Design review of the part built by this model. Coordinates are the model's own, in mm. A direction names the side the tool comes from. Coordinates: 2 decimals unless noted, no trailing zeros. Write each loop counter-clockwise with the first axis right and the second up, starting at its lowest first coordinate (ties: lowest second). Pieces come first, ordered by that corner, then holes. Notation, with made-up numbers: (-20.5, 72) - (29.5, 72) arc R25 cw to (29.5, 108) - close; hole circle Ø3 at (86.25, 12.5). An arc over 180 degrees is marked (long way). Use a Markdown table: item, result.
from build123d import *

# Parameters (mm, degrees)
SKETCH_W        = 37
SKETCH_H        = 37
PAD_DEPTH       = 17.8
SKETCH001_W     = 30.1
SKETCH001_H     = 30.1
POCKET_DEPTH    = 14.8
SKETCH002_R     = 1
PAD001_DEPTH    = 3.2
SKETCH003_W     = 31
SKETCH003_H     = 31
POCKET001_DEPTH = 10
SKETCH004_W     = 2.2
SKETCH004_H     = 1.6
POCKET002_DEPTH = 10
POCKET003_DEPTH = 2
POCKET004_DEPTH = 1.5
SKETCH011_W     = 8.94
SKETCH011_H     = 3.16
POCKET007_DEPTH = 3.5
SKETCH012_W     = 14.612
SKETCH012_H     = 7.87
POCKET008_DEPTH = 1.5
SKETCH013_W     = 7.7
SKETCH013_H     = 1.75
POCKET009_DEPTH = 3.5
PAD005_DEPTH    = 5
POCKET014_DEPTH = 2.1
SKETCH021_W     = 2.79
SKETCH021_H     = 4.318
POCKET013_DEPTH = 2.5
POCKET011_DEPTH = 3
POCKET012_DEPTH = 3.5
FILLET006_R     = 2
CHAMFER_SIZE    = 1
FILLET007_R     = 1
FILLET008_R     = 1


with BuildPart() as part:
    # Sketch → Pad (new body)
    with BuildSketch(Plane.XY):
        Rectangle(SKETCH_W, SKETCH_H)
    extrude(amount=PAD_DEPTH)

    # Sketch001 → Pocket (cut)
    with BuildSketch(Plane.XY):
        Rectangle(SKETCH001_W, SKETCH001_H)
    extrude(amount=POCKET_DEPTH, mode=Mode.SUBTRACT)

    # Sketch002 (on Face11 of Pocket) → Pad001 (join)
    with BuildSketch(Plane.XY.offset(14.8)):
        with Locations((1.018, 12.079)):
            Circle(SKETCH002_R)
        with Locations((9.384, -0.351)):
            Circle(SKETCH002_R)
        with Locations((-7.888, -4.939)):
            Circle(SKETCH002_R)
    extrude(amount=-PAD001_DEPTH)

    # Sketch003 → Pocket001 (cut)
    with BuildSketch(Plane.XY):
        Rectangle(SKETCH003_W, SKETCH003_H)
    extrude(amount=POCKET001_DEPTH, mode=Mode.SUBTRACT)

    # Sketch004 → Pocket002 (cut)
    with BuildSketch(Plane.XY):
        with Locations((-4.066, -15.8)):
            Rectangle(SKETCH004_W, SKETCH004_H)
    extrude(amount=POCKET002_DEPTH, mode=Mode.SUBTRACT)

    # Sketch005 (on Face16 of Pocket002) → Pocket003 (cut)
    with BuildSketch(Plane(origin=(0, -15.05, 0), x_dir=(-1, 0, 0), z_dir=(0, 1, 0))):
        with BuildLine():
            ThreePointArc((0.066, 14.4), (-2.134, 12.2), (0.066, 10))
            Line((0.066, 10), (6.566, 10))
            ThreePointArc((6.566, 10), (8.766, 12.2), (6.566, 14.4))
            Line((6.566, 14.4), (0.066, 14.4))
        make_face()
    extrude(amount=-POCKET003_DEPTH, mode=Mode.SUBTRACT)

    # Sketch006 (on Face18 of Pocket003) → Pocket004 (cut)
    with BuildSketch(Plane(origin=(0, -17.05, 0), x_dir=(-1, 0, 0), z_dir=(0, 1, 0))):
        with BuildLine():
            ThreePointArc((2.566, 14.3), (0.466, 12.2), (2.566, 10.1))
            Line((2.566, 10.1), (4.066, 10.1))
            ThreePointArc((4.066, 10.1), (6.166, 12.2), (4.066, 14.3))
            Line((4.066, 14.3), (2.566, 14.3))
        make_face()
    extrude(amount=-POCKET004_DEPTH, mode=Mode.SUBTRACT)

    # Sketch011 (on Face26 of Pocket004) → Pocket007 (cut)
    with BuildSketch(Plane.XZ.offset(-15.05)):
        with Locations((9.638, 13.18)):
            Rectangle(SKETCH011_W, SKETCH011_H)
    extrude(amount=-POCKET007_DEPTH, mode=Mode.SUBTRACT)

    # Sketch012 (on Face1 of Pocket007) → Pocket008 (cut)
    with BuildSketch(Plane(origin=(0, 18.5, 0), x_dir=(-1, 0, 0), z_dir=(0, 1, 0))):
        with Locations((-11.194, 13.865)):
            Rectangle(SKETCH012_W, SKETCH012_H)
    extrude(amount=-POCKET008_DEPTH, mode=Mode.SUBTRACT)

    # Sketch013 (on Face34 of Pocket008) → Pocket009 (cut)
    with BuildSketch(Plane(origin=(15.05, 0, 0), x_dir=(0, -1, 0), z_dir=(-1, 0, 0))):
        with Locations((-0.776, 12.425)):
            Rectangle(SKETCH013_W, SKETCH013_H)
    extrude(amount=-POCKET009_DEPTH, mode=Mode.SUBTRACT)

    # Sketch015 → Pad005 (join, symmetric)
    with BuildSketch(Plane.XZ):
        Polygon((-17, 0), (-18.5, 0), (-18.5, -3), (-19.3, -3), (-19.3, -3.5), (-18, -5), (-17, -5), align=None)
        Polygon((17, 0), (18.5, 0), (18.5, -3), (19.3, -3), (19.3, -3.5), (18, -5), (17, -5), align=None)
    extrude(amount=PAD005_DEPTH, both=True)

    # Sketch022 (on Face2 of Pad005) → Pocket014 (cut)
    with BuildSketch(Plane(origin=(0, 0, 0), x_dir=(1, 0, 0), z_dir=(0, 0, -1))):
        Polygon((-17.1, 17.1), (-11.9, 17.1), (-11.9, 15.5), (-15.5, 15.5), (-15.5, 11.9), (-17.1, 11.9), align=None)
        Polygon((17.1, 17.1), (11.9, 17.1), (11.9, 15.5), (15.5, 15.5), (15.5, 11.9), (17.1, 11.9), align=None)
        Polygon((-17.1, -17.1), (-11.9, -17.1), (-11.9, -15.5), (-15.5, -15.5), (-15.5, -11.9), (-17.1, -11.9), align=None)
        Polygon((17.1, -17.1), (11.9, -17.1), (11.9, -15.5), (15.5, -15.5), (15.5, -11.9), (17.1, -11.9), align=None)
    extrude(amount=-POCKET014_DEPTH, mode=Mode.SUBTRACT)

    # Sketch021 (on Face51 of Pad005) → Pocket013 (cut)
    with BuildSketch(Plane(origin=(0, 0, 14.8), x_dir=(1, 0, 0), z_dir=(0, 0, -1))):
        with Locations((-12.335, 12.686)):
            Rectangle(SKETCH021_W, SKETCH021_H)
    extrude(amount=-POCKET013_DEPTH, mode=Mode.SUBTRACT)

    # Sketch019 (on Face6 of Pocket013) → Pocket011 (cut)
    with BuildSketch(Plane.XY.offset(17.8)):
        with BuildLine():
            ThreePointArc((-5.133975, -2.5), (-6.5, -2.133975), (-6.866025, -3.5))
            Line((-6.866025, -3.5), (-2.247223, -11.5))
            ThreePointArc((-2.247223, -11.5), (-0.881198, -11.866025), (-0.515172, -10.5))
            Line((-0.515172, -10.5), (-5.133975, -2.5))
        make_face()
        with BuildLine():
            ThreePointArc((-0.133975, -2.5), (-1.5, -2.133975), (-1.866025, -3.5))
            Line((-1.866025, -3.5), (2.752777, -11.5))
            ThreePointArc((2.752777, -11.5), (4.118802, -11.866025), (4.484828, -10.5))
            Line((4.484828, -10.5), (-0.133975, -2.5))
        make_face()
        with BuildLine():
            ThreePointArc((4.866025, -2.5), (3.5, -2.133975), (3.133975, -3.5))
            Line((3.133975, -3.5), (7.752777, -11.5))
            ThreePointArc((7.752777, -11.5), (9.118802, -11.866025), (9.484828, -10.5))
            Line((9.484828, -10.5), (4.866025, -2.5))
        make_face()
        with BuildLine():
            ThreePointArc((9.866025, -2.5), (8.5, -2.133975), (8.133975, -3.5))
            Line((8.133975, -3.5), (12.752777, -11.5))
            ThreePointArc((12.752777, -11.5), (14.118802, -11.866025), (14.484828, -10.5))
            Line((14.484828, -10.5), (9.866025, -2.5))
        make_face()
    extrude(amount=-POCKET011_DEPTH, mode=Mode.SUBTRACT)

    # Sketch020 (on Face7 of Pocket011) → Pocket012 (cut)
    with BuildSketch(Plane(origin=(-18.5, 0, 0), x_dir=(0, -1, 0), z_dir=(-1, 0, 0))):
        Polygon((-2.464102, 14.6), (1, 14.6), (-0.732051, 11.6), align=None)
        Polygon((-7.464102, 14.6), (-4, 14.6), (-5.732051, 11.6), align=None)
        Polygon((-12.464102, 14.6), (-9, 14.6), (-10.732051, 11.6), align=None)
    extrude(amount=-POCKET012_DEPTH, mode=Mode.SUBTRACT)

    # Fillet006
    fillet006_edges = [part.edges().sort_by_distance(p)[0] for p in [
        (11.194, 17, 17.8),
        (3.888, 17.75, 17.8),
        (-7.306, 18.5, 17.8),
        (18.5, -0.75, 17.8),
        (18.5, 17, 13.865),
        (18.5, 17.75, 9.93),
        (18.5, 18.5, 4.965),
        (-18.5, 18.5, 8.9),
        (-18.5, 0, 17.8),
        (-18.5, -18.5, 8.9),
        (0, -18.5, 17.8),
        (18.5, -18.5, 8.9),
    ]]
    fillet(fillet006_edges, radius=FILLET006_R)

    # Chamfer
    chamfer_edges = [part.edges().sort_by_distance(p)[0] for p in [
        (-3.316, -18.5, 14.3),
    ]]
    chamfer(chamfer_edges, length=CHAMFER_SIZE)

    # Fillet007
    fillet007_edges = [part.edges().sort_by_distance(p)[0] for p in [
        (10.194, 18.5, 9.93),
        (3.888, 18.5, 12.865),
        (5.168, 17, 13.18),
        (9.638, 17, 11.6),
        (14.108, 17, 13.18),
        (9.638, 17, 14.76),
        (3.180098, 17.792098, 17.326592),
        (18.026592, 17.792098, 9.222098),
    ]]
    fillet(fillet007_edges, radius=FILLET007_R)

    # Fillet008
    fillet008_edges = [part.edges().sort_by_distance(p)[0] for p in [
        (18.5, 0.776, 13.3),
        (18.5, -3.074, 12.425),
        (18.5, 0.776, 11.55),
        (18.5, 4.626, 12.425),
    ]]
    fillet(fillet008_edges, radius=FILLET008_R)


solid = part.part
(1) For L1, parallel to Y at x = 1, z = 12; L2, parallel to X at y = 11, z = 5.75; L3, parallel to Y at x = 11.5, z = 10.75, list the stretches that pass through material, from the lowest coordinate up. Write a range as from..to.
Determined:
| item | result |
|---|---|
| L1 | -18.5..-17.05, 11.08..13.08, 15.05..18.5 |
| L2 | -18.5..-15.5, 15.5..18.5 |
| L3 | -18.5..-15.05, 15.05..16.99 |
(2) Machinability: for faces 1 (the flat face through (-16.8, 1.6, 13.1)), 2 (the cylindrical face through (3.6, 18.2, 12.4)), 3 (the cylindrical face through (-0.467, -17.272, 12.246)), 4 (the flat face through (-12, -14.845, 16)), which of the approach directions +Z, -Z, +X, -X, +Y, -Y give a long, thin tool a straight path to every point of the face, cutting with its end or side? Answer none if there is none.
Determined:
| item | result |
|---|---|
| face 1 | -X |
| face 2 | +Z, +X, +Y |
| face 3 | -Y |
| face 4 | -Z |
(3) Draft analysis for pull direction Z (two halves, no side actions). For faces 5 (the cylindrical face through (2.133, -16.036, 12.248)), 6 (the flat face through (17.5, -0.1, -5)), 7 (the flat face through (-17.1, -14, 1)), state which applies: +Z half, -Z half, draft (parallel to the pull), parting line (faces both ways), or undercut.
Determined:
| item | result |
|---|---|
| face 5 | undercut |
| face 6 | -Z half |
| face 7 | draft |
(4) Take a section at B-B on x = -14.5. Write out the cut boundary in (y, z).
Determined:
| item | result |
|---|---|
| outline | (-18.5, 0) - (-17.1, 0) - (-17.1, 2.1) - (-15.5, 2.1) - (-15.5, 10) - (-15.05, 10) - (-15.05, 14.8) - (15.05, 14.8) - (15.05, 10) - (15.5, 10) - (15.5, 2.1) - (17.1, 2.1) - (17.1, 0) - (18.5, 0) - (18.5, 15.8) arc R2 ccw to (16.5, 17.8) - (-16.5, 17.8) arc R2 ccw to (-18.5, 15.8) - close |
(5) For pin 1 (0.6 mm diameter, centred on x = 1, y = 11.5, fed in from -Z); pin 2 (1.4 mm diameter, centred on x = -12, y = -11.5, fed in from -Z); pin 3 (2 mm diameter, centred on y = -5.5, z = 11, fed in from -X), all flat-tipped, find the tip position at first contact; note any pin that passes through.
Determined:
| item | result |
|---|---|
| pin 1 | z = 11.6 |
| pin 2 | z = 17.3 |
| pin 3 | x = -18.5 |
(6) Take a section at A-A on y = -10. State how many separate pieces and enclosed holes the cut face has, and give its area (3 significant figures).
Determined:
| item | result |
|---|---|
| separate pieces | 5 |
| enclosed holes | 0 |
| area | 175 mm2 |
